Verification items for the finished model (mm, model axes). A direction names the side the tool comes from. Round coordinates to 2 decimals unless told otherwise and drop trailing zeros. Order: outer loops, then holes, each group sorted by start corner. A loop starts at its lowest first (then second) coordinate and runs counter-clockwise, first axis right, second up. Notation, with made-up numbers: (-29.75, 15.25) -> (-21.75, 15.25) arc R30 ccw to (-21.75, 39.25) -> close; hole circle Ø9 at (-34, 70). An arc over 180 degrees is marked (long way). Return JSON: item names as keys, results as strings. Group by question number.
1) Depth check by flat-ended pin: pin 1 (4 mm diameter, centred on x = 10.5, z = -18.19, fed in from -Y); pin 2 (6 mm diameter, centred on y = 10.5, z = -27, fed in from -X); pin 3 (10.5 mm diameter, centred on x = -67.5, z = 0, fed in from -Y); pin 4 (1 mm diameter, centred on x = 34, y = 34.5, fed in from +Z). Enter the tip coordinate at first touch or a pass-through.
2) Section check A-A on y = 22. Enter the section's corners in (x, z).
3) Scan lines: L1, parallel to Z at x = -47.5, y = 8.5; L2, parallel to X at y = 18.25, z = 0; L3, parallel to X at y = 46, z = 0. Record each from-to range of solid material in increasing order.
4) Section check B-B on x = 67.5. Enter the section's corners in (y, z), plus the area to 3 significant figures.
5) Section check C-C on x = 2. State how many separate pieces and enclosed holes the cut face has, plus the area to 3 significant figures.
6) Tool access check on faces 3 (the cylindrical face through (12.94, 44.93, 17.64)), 4 (the cylindrical face through (-47.906, 7.605, -43.734)), 5 (the flat face through (-8, 38, -16)). Record the directions out of +Z, -Z, +X, -X, +Y, -Y that give a thin tool (end or side, any length) a straight path to the whole face; none if there is none.
7) Draft check along X on faces 1 (the conical face through (25.039, 48.749, 7.885)), 2 (the conical face through (-10.37, 38.76, -17.77)). Enter one of: pulls with the +X half, pulls with the -X half, needs draft (parallel to the pull), parting line crosses it, or undercut.
Autodesk Inventor part; units mm, degrees
ref_plane "Work Plane1" through (45, 0, 0) normal (1, 0, 0) x (0, 1, 0)
ref_plane "XZ Plane" through (0, 0, 0) normal (0, 1, 0) x (-1, 0, 0)
ref_plane "XY Plane" through (0, 0, 0) normal (0, 0, 1) x (1, 0, 0)
sketch "Sketch1" plane through (0, 0, 0) normal (0, 0, 1) x (1, 0, 0)
  line L0 (0, 0) -> (0, 50)
  line L1 (45, 0) -> (75, 0)
  line L2 (75, 0) -> (75, 15)
  line L3 (75, 15) -> (45, 15)
  line L4 (45, 15) -> (45, 50)
  line L5 (45, 50) -> (0, 50)
  line L6 (0, 50) -> (0, 38)
  line L7 (45, 0) -> (45, 10)
  line L8 (45, 10) -> (35, 10)
  line L9 (35, 10) -> (35, 38)
  line L10 (35, 38) -> (0, 38)
  line L11 (0, 0) -> (35, 0)
  line L12 (45, 0) -> (45, 0)
  dimension "d1" = 50
  dimension "d2" = 15
  dimension "d4" = 12
  dimension "d5" = 10
  dimension "d6" = 150
  dimension "d7" = 90
  dimension "d8" = 70
  dimension "d9" = 10
revolve "Revolution1" add sketch "Sketch1" angle 360 about axis through (0, 0, 0) along (0, 1, 0)
chamfer "Chamfer1" distance 20 angle 45 1 edges at (-45, 50, 0)
ref_plane "Work Plane1" through (45, 0, 0) normal (1, 0, 0) x (0, 1, 0)
sketch "Sketch4" plane through (45, 0, 0) normal (1, 0, 0) x (0, 1, 0)
  circle A0 centre (44.772, 0) radius 6.35
  point P0 (0, 0)
  dimension "d22" = 12.7
sketch "Sketch5" plane through (0, 0, 0) normal (0, 0, 1) x (1, 0, 0)
  line L0 (44.9751, 46.9317) -> (33.3301, 30)
  line L1 (45, 30) -> (-45, 30)
  point P0 (0, 0)
sweep "Sweep3" cut profiles "Sketch4" path "Sketch5" path curves L0
sketch "Sketch6" plane through (0, 50, 0) normal (0, 1, 0) x (1, 0, 0)
  circle A0 centre (0, 0) radius 17.5
  dimension "d25" = 35
hole "Hole1" at (0, 50, 0) direction (0, -1, 0) diameter 35 depth 15 tip angle 118
sketch "Sketch7" plane through (0, 50, 0) normal (0, 1, 0) x (1, 0, 0)
  circle A0 centre (-21, 0) radius 2.75
  circle A1 centre (-10.5, -18.1865) radius 2.75
  circle A2 centre (10.5, -18.1865) radius 2.75
  circle A3 centre (21, 0) radius 2.75
  circle A4 centre (10.5, 18.1865) radius 2.75
  circle A5 centre (-10.5, 18.1865) radius 2.75
  point P0 (0, 0)
  dimension "d34" = 5.5
  dimension "d37" = 360
  dimension "d58" = 21
hole "Hole2" at (-10.5, 50, -18.1865) at (10.5, 50, -18.1865) at (21, 50, 0) at (10.5, 50, 18.1865) at (-10.5, 50, 18.1865) at (-21, 50, 0) direction (0, -1, 0) diameter 5 depth 10 tip angle 118
thread "Thread1"
thread "Thread2"
thread "Thread3"
thread "Thread4"
thread "Thread5"
thread "Thread6"
sketch "Sketch8" plane through (0, 15, 0) normal (0, 1, 0) x (1, 0, 0)
  point P0 (0, 0)
sketch "Sketch9" plane through (0, 0, 0) normal (0, -1, 0) x (1, 0, 0)
  point P0 (0, 0)
sketch "Sketch10" plane through (0, 0, 0) normal (0, -1, 0) x (1, 0, 0)
  point P0 (0, 0)
sketch "Sketch11" plane through (0, 0, 0) normal (0, -1, 0) x (1, 0, 0)
  circle A0 centre (0, 0) radius 17.5
  circle A1 centre (0, 0) radius 67.5 construction
  circle A2 centre (67.5, 0) radius 4
  circle A3 centre (47.7297, -47.7297) radius 4
  circle A4 centre (0, -67.5) radius 4
  circle A5 centre (-47.7297, -47.7297) radius 4
  circle A6 centre (-67.5, 0) radius 4
  circle A7 centre (-47.7297, 47.7297) radius 4
  circle A8 centre (0, 67.5) radius 4
  circle A9 centre (47.7297, 47.7297) radius 4
  dimension "d59" = 135
  dimension "d60" = 8
  dimension "d94" = 360
hole "Hole3" at (67.5, 0, 0) direction (0, 1, 0) diameter 8 end through all
hole "Hole4" at (47.7297, 0, 47.7297) at (0, 0, 67.5) at (-47.7297, 0, 47.7297) at (-67.5, 0, 0) at (-47.7297, 0, -47.7297) at (0, 0, -67.5) at (47.7297, 0, -47.7297) direction (0, 1, 0) diameter 8 end through all
properties part number "final injector body" material "Stainless Steel"
Check result:
{
 "1": {"pin 1": "y = 38", "pin 2": "x = -71.06", "pin 3": "y = 0", "pin 4": "z = 23.18"},
 "2": {"outline": "circle Ø90 at (0, 0); hole circle Ø70 at (0, 0)"},
 "3": {"L1": "-58.04 to -51.72, -43.74 to 43.74, 51.72 to 58.04", "L2": "-45 to -35, 35 to 45", "L3": "-29 to -23.5, -18.5 to -17.5, 17.5 to 18.5, 23.5 to 29"},
 "4": {"outline": "(0, -32.69) -> (15, -32.69) -> (15, -4) -> (0, -4) -> close; (0, 4) -> (15, 4) -> (15, 32.69) -> (0, 32.69) -> close", "area": "861 mm^2"},
 "5": {"separate pieces": "4", "enclosed holes": "0", "area": "1,510 mm^2"},
 "6": {"face 3": "+Y", "face 4": "+Y, -Y", "face 5": "-Y"},
 "7": {"face 1": "parting line crosses it", "face 2": "undercut"}
}
